Could you check a few things on this model? Use its own coordinates, in mm. A direction names the side the tool comes from. Coordinates: 2 decimals unless noted, no trailing zeros. Order: outer loops, then holes, each group sorted by start corner. A loop starts at its lowest first (then second) coordinate and runs counter-clockwise, first axis right, second up. Notation, with made-up numbers: (31.5, 21) -> (89.5, 21) arc R19 cw to (89.5, 47) -> close; hole circle Ø1 at (85, -28). An arc over 180 degrees is marked (long way). Use a Markdown table: item, result. Add a question column.
1) If we section it at C-C (x = 3.75): Write out the boundary of the cut face in (y, z).
2) If we section it at A-A (y = 47): Write out the boundary of the cut face in (x, z), plus the area to 3 significant figures.
3) Which directions (+Z, -Z, +X, -X, +Y, -Y) give clear straight access to the entire face, cutting with the end or side of a thin tool? Please do faces 1 (the flat face through (5, 19, 110)), 2 (the flat face through (5, 100, 2)).
4) Will this pin go through, and if not, where does the flat tip stop? pin 1 Ø1 at (y, z) = (-68.5, 102) entering from -X.
5) If we section it at B-B (z = 81): Write out the boundary of the cut face in (x, y).
6) If I drill on L1, parallel to Z at x = 2.25, y = 39.5; L2, parallel to Y at x = 5.75, z = 87; L3, parallel to Y at x = 6, z = -120, over which ranges is the centre line in solid material (lowest first)? Write a range as [from, to].
```python
from build123d import *

# Parameters (mm, degrees)
SKETCH1_W           = 300
SKETCH1_H           = 200
BOSS_EXTRUDE1_DEPTH = 10
SKETCH2_R           = 2
SKETCH2_R_2         = 4
CUT_EXTRUDE1_DEPTH  = 10
SKETCH3_W           = 80
SKETCH3_H           = 80
CUT_EXTRUDE2_DEPTH  = 10


with BuildPart() as part:
    # Sketch1 → Boss-Extrude1 (new body)
    with BuildSketch(Plane(origin=(0, 0, 0), x_dir=(0, 0, -1), z_dir=(1, 0, 0))):
        Rectangle(SKETCH1_W, SKETCH1_H)
    extrude(amount=BOSS_EXTRUDE1_DEPTH)

    # Sketch2 → Cut-Extrude1 (cut)
    with BuildSketch(Plane(origin=(10, 0, 0), x_dir=(0, 0, -1), z_dir=(1, 0, 0))):
        with Locations((120, 70)):
            Circle(SKETCH2_R)
        with Locations((56.786077483, 60)):
            Circle(SKETCH2_R_2)
    extrude(amount=-CUT_EXTRUDE1_DEPTH, mode=Mode.SUBTRACT)

    # Sketch3 → Cut-Extrude2 (cut)
    with BuildSketch(Plane(origin=(10, 0, 0), x_dir=(0, 0, -1), z_dir=(1, 0, 0))):
        with Locations((-70, 20)):
            Rectangle(SKETCH3_W, SKETCH3_H)
    extrude(amount=-CUT_EXTRUDE2_DEPTH, mode=Mode.SUBTRACT)


solid = part.part
```
Answer sheet:
| question | item | result |
|---|---|---|
| 1 | outline | (-100, -150) -> (100, -150) -> (100, 150) -> (-100, 150) -> close; hole (-20, 30) -> (60, 30) -> (60, 110) -> (-20, 110) -> close; hole circle Ø8 at (60, -56.79); hole circle Ø4 at (70, -120) |
| 2 | outline | (0, -150) -> (10, -150) -> (10, 30) -> (0, 30) -> close; (0, 110) -> (10, 110) -> (10, 150) -> (0, 150) -> close |
| 2 | area | 2,200 mm2 |
| 3 | face 1 | +X, -X |
| 3 | face 2 | +Z, -Z, +X, -X, +Y |
| 4 | pin 1 | x = 0 |
| 5 | outline | (0, -100) -> (10, -100) -> (10, -20) -> (0, -20) -> close; (0, 60) -> (10, 60) -> (10, 100) -> (0, 100) -> close |
| 6 | L1 | [-150, 30], [110, 150] |
| 6 | L2 | [-100, -20], [60, 100] |
| 6 | L3 | [-100, 68], [72, 100] |
